Here's how the part is built. I have some questions about the finished solid (model axes, mm). Face numbers are marked on the shaded views. A direction names the side the tool comes from. Round coordinates to 2 decimals unless told otherwise and drop trailing zeros. Write each loop counter-clockwise with the first axis right and the second up, starting at its lowest first coordinate (ties: lowest second). Pieces come first, ordered by that corner, then holes. Notation, with made-up numbers: (66, 2) -> (91, 2) arc R11 cw to (91, 15) -> close; hole circle Ø6 at (6.5, 0). An arc over 180 degrees is marked (long way). Answer as CSV lines item,"result".
```python
from build123d import *

# Parameters (mm, degrees)
BOSS_EXTRUDE1_DEPTH = 8.5
SKETCH2_W           = 17
SKETCH2_H           = 17
CUT_EXTRUDE1_DEPTH  = 6
CUT_EXTRUDE2_DEPTH  = 3
BOSS_EXTRUDE2_DEPTH = 1


with BuildPart() as part:
    # Sketch1 → Boss-Extrude1 (new body, symmetric)
    with BuildSketch(Plane(origin=(0, 0, 0), x_dir=(0, 0, -1), z_dir=(1, 0, 0))):
        Polygon((0, 0), (-20, 0), (-20, -3), (-11.5, -11.5), (-3, -20), (0, -20), align=None)
    extrude(amount=BOSS_EXTRUDE1_DEPTH, both=True)

    # Sketch2 → Cut-Extrude1 (cut, symmetric)
    with BuildSketch(Plane(origin=(0, 0, 0), x_dir=(0, 0, -1), z_dir=(1, 0, 0))):
        with Locations((-11.5, -11.5)):
            Rectangle(SKETCH2_W, SKETCH2_H)
    extrude(amount=CUT_EXTRUDE1_DEPTH, both=True, mode=Mode.SUBTRACT)

    # Sketch3 → Cut-Extrude2 (cut)
    with BuildSketch(Plane.XY.offset(3)):
        with BuildLine():
            Line((-3, -9), (-3, -12))
            ThreePointArc((-3, -12), (0, -15), (3, -12))
            Line((3, -12), (3, -9))
            ThreePointArc((3, -9), (0, -6), (-3, -9))
        make_face()
    cut_extrude2 = extrude(amount=-CUT_EXTRUDE2_DEPTH, mode=Mode.SUBTRACT)

    # Sketch4 → Boss-Extrude2 (add)
    with BuildSketch(Plane(origin=(0, 0, 0), x_dir=(-1, 0, 0), z_dir=(0, 0, -1))):
        with BuildLine():
            Line((-1, -3), (1, -3))
            ThreePointArc((1, -3), (1.85, -2.15), (1, -1.3))
            Line((1, -1.3), (-1, -1.3))
            ThreePointArc((-1, -1.3), (-1.85, -2.15), (-1, -3))
        make_face()
        with BuildLine():
            Line((-1, -18.3), (1, -18.3))
            ThreePointArc((1, -18.3), (1.85, -17.45), (1, -16.6))
            Line((1, -16.6), (-1, -16.6))
            ThreePointArc((-1, -16.6), (-1.85, -17.45), (-1, -18.3))
        make_face()
    boss_extrude2 = extrude(amount=BOSS_EXTRUDE2_DEPTH)

    # Mirror1: Cut-Extrude2, Boss-Extrude2 across plane
    add(cut_extrude2.mirror(Plane(origin=(0, 0, 0), x_dir=(0, -0.707106781, 0.707106781), z_dir=(0, 0.707106781, 0.707106781))), mode=Mode.SUBTRACT)
    add(boss_extrude2.mirror(Plane(origin=(0, 0, 0), x_dir=(0, -0.707106781, 0.707106781), z_dir=(0, 0.707106781, 0.707106781))))


solid = part.part
```
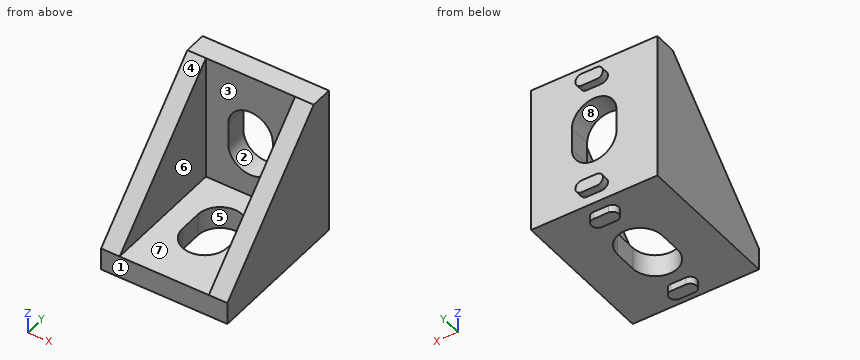
1. On a 3-axis mill with a long thin cutter (end or side, diameter ignored), from which of +Z, -Z, +X, -X, +Y, -Y can I reach the whole of each face in a straight line? I mean the marked faces 1, 2, 3, 4 and 5. Say none if no direction works.
Numbers:
face 1,"+Z, -Z, +X, -X, -Y"
face 2,"+Y, -Y"
face 3,"+Z, -Y"
face 4,"+Z, +X, -X, -Y"
face 5,"+Z, -Z"
2. Suppose I cut it at B-B on z = 2.15. Please give me the cut outline in (x, y), and give its area (3 significant figures).
Numbers:
outline,"(-8.5, -20) -> (8.5, -20) -> (8.5, 0) -> (1.85, 0) -> (1.85, 1) -> (-1.85, 1) -> (-1.85, 0) -> (-8.5, 0) -> close; hole (-3, -12) arc R3 ccw to (3, -12) -> (3, -9) arc R3 ccw to (-3, -9) -> close"
area,"297 mm^2"
3. For pin 1 Ø6 at (x, y) = (4.5, -5.5) entering from +Z; pin 2 Ø0.8 at (x, z) = (0.5, -0.5) entering from +Y; pin 3 Ø1.1 at (x, y) = (-0.5, 0.5) entering from -Z; pin 4 Ø0.8 at (x, y) = (0.5, 0.5) entering from +Z, each with a flat end and sliding along its axis, tell me the tip position at first contact or that it passes through.
Numbers:
pin 1,"stops at z = 20"
pin 2,"stops at y = -1.3"
pin 3,"stops at z = 0"
pin 4,"stops at z = 18.3"
4. Suppose I cut it at A-A on y = -11.5. Please give me the cut outline in (x, z).
Numbers:
outline,"(-8.5, 0) -> (-3, 0) -> (-3, 3) -> (-6, 3) -> (-6, 11.5) -> (-8.5, 11.5) -> close; (3, 0) -> (8.5, 0) -> (8.5, 11.5) -> (6, 11.5) -> (6, 3) -> (3, 3) -> close"
5. If I drill on line 1 (X direction, y = -4, z = 7.25); line 2 (Y direction, x = -4.75, z = 10); line 3 (Z direction, x = -7, y = -0.5), over which ranges is the centre line in solid material (lowest first)?
Numbers:
line 1,"x = -8.5 to -6, 6 to 8.5"
line 2,"y = -3 to 0"
line 3,"z = 0 to 20"
6. If we mould it in two halves opening along Z, with no side actions, what happens to the marked faces 6, 7 and 8? For each: released by +Z, released by -Z, zero draft, split by the parting line, or undercut.
Numbers:
face 6,"zero draft"
face 7,"released by +Z"
face 8,"undercut"
7. Suppose I cut it at C-C on x = 0. Count the separate pieces of the cut face and the enclosed holes in it, and give its area (3 significant figures).
Numbers:
separate pieces,"3"
enclosed holes,"0"
area,"63.8 mm^2"
8. Suppose I cut it at D-D on y = -0.5. Please give me the cut outline in (x, z), and give its area (3 significant figures).
Numbers:
outline,"(-8.5, 0) -> (8.5, 0) -> (8.5, 20) -> (-8.5, 20) -> close; hole (-3, 9) arc R3 ccw to (3, 9) -> (3, 12) arc R3 ccw to (-3, 12) -> close"
area,"294 mm^2"
